Check sheet for the modelled part. Datum: model origin and axes. Units: mm. A direction names the side the tool comes from. Give positions to 0.01 mm unless a question says otherwise; leave off trailing zeros. Loops run counter-clockwise (first coordinate to the right, second up) from the corner with the lowest first, then second, coordinate; pieces in that order, holes last. Notation, with made-up numbers: (84.5, 83.5) -> (105.5, 83.5) arc R25 cw to (105.5, 100.5) -> close; hole circle Ø9 at (66, 51.5). An arc over 180 degrees is marked (long way). Write each question's results on one line, items separated by ' | '. Start each with the question number.
Item 1: Cross-section at B-B on y = 0.6. State how many separate pieces and enclosed holes the cut face has, then the cut area to 3 significant figures.
Item 2: Scan lines: line 1 along X through (y, z) = (2.2, -5); line 2 along Z through (x, y) = (14, 0.45); line 3 along Z through (x, y) = (7, 0.6). Record each from-to range of solid material in increasing order.
Item 3: Gauge pin test, flat ends, axial feed: pin 1 Ø1 at (x, y) = (47.5, 1.5) entering from +Z; pin 2 Ø1.6 at (y, z) = (1, 27) entering from -X; pin 3 Ø1 at (y, z) = (1, 27) entering from +X. Record the tip position at first contact, or that the pin passes through.
Item 4: Cross-section at C-C on x = -32.5. Enter the section's corners in (y, z) (3 decimals).
Item 5: Mould release check, pull along Z, two halves, no side actions. Record for faces 4 (the face through (15, 2, -3.35)), 5 (the face through (17.33, 2, -5)), 6 (the face through (-36.667, 2, 27)), 7 (the face through (-1, 2, -25)): pulls with the +Z half, pulls with the -Z half, needs draft (parallel to the pull), parting line crosses it, or undercut.
Item 6: Access from +Z, -Z, +X, -X, +Y, -Y to the whole of each face (thin tool, end or side, straight path). Record for faces 1 (the face through (-20, 2, 27)), 2 (the face through (15, 2, -6.65)), 3 (the face through (48, 2, 25)).
Item 7: Cross-section at A-A on z = -4.5. Enter the section's corners in (x, y) (3 decimals), then the cut area to 3 significant figures.
from build123d import *

# Parameters (mm, degrees)
BOSS_EXTRUDE1_DEPTH = 3.175
SKETCH2_W           = 5
SKETCH2_H           = 3.3
CUT_EXTRUDE1_DEPTH  = 3.175


with BuildPart() as part:
    # Sketch1 → Boss-Extrude1 (new body)
    with BuildSketch(Plane(origin=(0, 0, 0), x_dir=(1, 0, 0), z_dir=(0, 1, 0))):
        Polygon((-50, 25), (50, 25), (50, -25), (46.666666667, -25), (46.666666667, -28.175), (36.666666667, -28.175), (36.666666667, -25), (30, -25), (30, -28.175), (20, -28.175), (20, -25), (-20, -25), (-20, -28.175), (-30, -28.175), (-30, -25), (-36.666666667, -25), (-36.666666667, -28.175), (-46.666666667, -28.175), (-46.666666667, -25), (-50, -25), align=None)
    extrude(amount=BOSS_EXTRUDE1_DEPTH)

    # Sketch2 → Cut-Extrude1 (cut)
    with BuildSketch(Plane(origin=(0, 3.175, 0), x_dir=(1, 0, 0), z_dir=(0, 1, 0))):
        with Locations((-0.169597497, 5)):
            Rectangle(SKETCH2_W, SKETCH2_H)
        with Locations((-15.169597497, 5)):
            Rectangle(SKETCH2_W, SKETCH2_H)
        with Locations((14.830402503, 5)):
            Rectangle(SKETCH2_W, SKETCH2_H)
    extrude(amount=-CUT_EXTRUDE1_DEPTH, mode=Mode.SUBTRACT)


solid = part.part
Answer sheet:
1) separate pieces: 1 | enclosed holes: 3 | area: 5,080 mm²
2) line 1: x = -50 to -17.67, -12.67 to -2.67, 2.33 to 12.33, 17.33 to 50 | line 2: z = -25 to -6.65, -3.35 to 25 | line 3: z = -25 to 25
3) pin 1: stops at z = 25 | pin 2: stops at x = -46.67 | pin 3: stops at x = 46.67
4) outline: (0, -25) -> (3.175, -25) -> (3.175, 25) -> (0, 25) -> close
5) face 4: undercut | face 5: undercut | face 6: needs draft | face 7: pulls with the -Z half
6) face 1: +Z, +Y, -Y | face 2: +Y, -Y | face 3: +Z, +X, +Y, -Y
7) outline: (-50, 0) -> (-17.67, 0) -> (-17.67, 3.175) -> (-50, 3.175) -> close; (-12.67, 0) -> (-2.67, 0) -> (-2.67, 3.175) -> (-12.67, 3.175) -> close; (2.33, 0) -> (12.33, 0) -> (12.33, 3.175) -> (2.33, 3.175) -> close; (17.33, 0) -> (50, 0) -> (50, 3.175) -> (17.33, 3.175) -> close | area: 270 mm²
